The drawing under review shows one solid part. Ordinate dimensions are in mm from its lowest x, y, z. A direction names the side the tool comes from. Give positions to 0.01 mm unless a question says otherwise; leave off trailing zeros. Order: outer loops, then holes, each group sorted by start corner. A loop starts at its lowest first (then second) coordinate and runs counter-clockwise, first axis right, second up. Notation, with made-up numbers: (80, 67.5) - (91, 67.5) arc R13 ccw to (91, 78.5) - close; hole circle Ø7 at (14, -12.75). An arc over 180 degrees is marked (long way). Use CSV: the item, a comma, the result in double quotes. Start each with the question number.
1. Take a section at B-B, the plane y = 5.25. State the section outline as (x, z) points.
2. Take a section at A-A, the plane x = 25. State the section outline as (y, z) points.
3. Take a section at C-C, the plane y = 10.25. State the section outline as (x, z) points, then the cut area to 3 significant figures.
4. Machinability: for the marked faces 4 and 5, which of the approach directions +Z, -Z, +X, -X, +Y, -Y give a long, thin tool a straight path to every point of the face, cutting with its end or side? Answer none if there is none.
5. Take a section at D-D, the plane z = 0.65. State the section outline as (x, y) points, then the cut area to 3 significant figures.
6. Draft analysis for pull direction Y (two halves, no side actions). For the marked faces 1, 2 and 3, state which applies: released by +Y, released by -Y, zero draft, split by the parting line, or undercut.
7. To check wall thickness, follow line 1 (Y direction, x = 10, z = 1.9); line 2 (X direction, y = 5.5, z = 1.2); line 3 (X direction, y = 1.75, z = 3.3). State the ranges of each line that lie inside material, in increasing order. Write a range as [from, to].
8. For pin 1 (1.1 mm diameter, centred on x = 0.5, z = 0.5, fed in from -Y); pin 2 (0.8 mm diameter, centred on x = 0.5, z = 4.5, fed in from +Y); pin 3 (4 mm diameter, centred on x = 22.5, y = 8.5, fed in from +Z), all flat-tipped, find the tip position at first contact; note any pin that passes through.
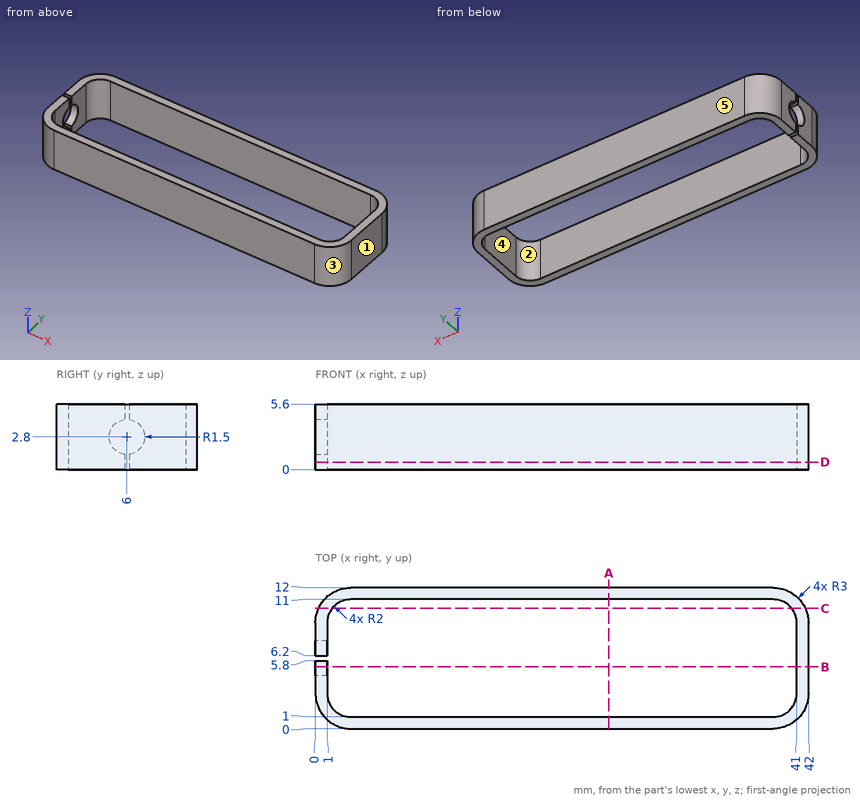
Determined:
1,outline,"(0, 0) - (1, 0) - (1, 1.5) - (0, 1.5) - close; (0, 4.1) - (1, 4.1) - (1, 5.6) - (0, 5.6) - close; (41, 0) - (42, 0) - (42, 5.6) - (41, 5.6) - close"
2,outline,"(0, 0) - (1, 0) - (1, 5.6) - (0, 5.6) - close; (11, 0) - (12, 0) - (12, 5.6) - (11, 5.6) - close"
3,outline,"(0.27, 0) - (1.44, 0) - (1.44, 5.6) - (0.27, 5.6) - close; (40.56, 0) - (41.73, 0) - (41.73, 5.6) - (40.56, 5.6) - close"
3,area,"13.1 mm²"
4,face 4,"+Z, -Z"
4,face 5,"+Z, -Z, +X, -X, +Y"
5,outline,"(0, 3) arc R3 ccw to (3, 0) - (39, 0) arc R3 ccw to (42, 3) - (42, 9) arc R3 ccw to (39, 12) - (3, 12) arc R3 ccw to (0, 9) - (0, 6.2) - (1, 6.2) - (1, 9) arc R2 cw to (3, 11) - (39, 11) arc R2 cw to (41, 9) - (41, 3) arc R2 cw to (39, 1) - (3, 1) arc R2 cw to (1, 3) - (1, 5.8) - (0, 5.8) - close"
5,area,"99.3 mm²"
6,face 1,"zero draft"
6,face 2,"undercut"
6,face 3,"released by -Y"
7,line 1,"y = [0, 1], [11, 12]"
7,line 2,"x = [0, 1], [41, 42]"
7,line 3,"x = [0.27, 1.44], [40.56, 41.73]"
8,pin 1,"stops at y = 0.72"
8,pin 2,"stops at y = 11.14"
8,pin 3,"passes through"
